from build123d import *

# Parameters (mm, degrees)
F0_W      = 31.75
F0_H      = 25.4
F0_R      = 3.175
F1_DEPTH  = 3.81
F2_W      = 31.75
F2_H      = 3.81
F3_DEPTH  = 25.4
F4_W      = 2.54
F4_H      = 25.4
F5_DEPTH  = 10.16
F4_W_2    = 8.89
F4_H_2    = 8.89
F6_DEPTH  = 25.4
F8_W      = 3.175
F8_H      = 25.4
F9_DEPTH  = 6.35
F7_W      = 3.18363
F7_H      = 25.4
F10_DEPTH = 6.35


with BuildPart() as f1:
    # F0 (on Top) → F1 (new body)
    with BuildSketch(Plane.XY):
        with Locations((-11.662145, 29.340504)):
            Rectangle(F0_W, F0_H)
        with Locations((-11.662145, 31.880504)):
            Circle(F0_R, mode=Mode.SUBTRACT)
    extrude(amount=F1_DEPTH)

    # F2 (on face) → F3 (join)
    with BuildSketch(Plane.XY.offset(3.81)):
        with Locations((-11.662145, 18.545504)):
            Rectangle(F2_W, F2_H)
    extrude(amount=F3_DEPTH)

    # F4 (on face) → F5 (join)
    with BuildSketch(Plane(origin=(0, 20.450504, 0), x_dir=(-1, 0, 0), z_dir=(0, 1, 0))):
        with Locations((-2.942855, 16.51)):
            Rectangle(F4_W, F4_H)
        with Locations((26.267145, 16.51)):
            Rectangle(F4_W, F4_H)
    extrude(amount=F5_DEPTH)

    # F4 (on face) → F6 (cut)
    with BuildSketch(Plane(origin=(0, 20.450504, 0), x_dir=(-1, 0, 0), z_dir=(0, 1, 0))):
        with Locations((11.662145, 18.415)):
            Rectangle(F4_W_2, F4_H_2)
    extrude(amount=-F6_DEPTH, mode=Mode.SUBTRACT)

    # F8 (on face) → F9 (join)
    with BuildSketch(Plane(origin=(1.672855, 0, 0), x_dir=(0, -1, 0), z_dir=(-1, 0, 0))):
        with Locations((-29.023004, 16.51)):
            Rectangle(F8_W, F8_H)
    extrude(amount=F9_DEPTH)

    # F7 (on face) → F10 (join)
    with BuildSketch(Plane.YZ.offset(-24.997145)):
        with Locations((29.018689, 16.51)):
            Rectangle(F7_W, F7_H)
    extrude(amount=F10_DEPTH)


solid = f1.part
Here's how the part is built. I have some questions about the finished solid (model axes, mm). A direction names the side the tool comes from. Round coordinates to 2 decimals unless told otherwise and drop trailing zeros. Loops run counter-clockwise (first coordinate to the right, second up) from the corner with the lowest first, then second, coordinate; pieces in that order, holes last.
1. If we section it at A-A on z = 17.5: Write out the boundary of the cut face in (x, y).
Answer list:
outline: (-27.54, 16.64) - (-16.11, 16.64) - (-16.11, 20.45) - (-25, 20.45) - (-25, 27.43) - (-18.65, 27.43) - (-18.65, 30.61) - (-27.54, 30.61) - close; (-7.22, 16.64) - (4.21, 16.64) - (4.21, 30.61) - (-4.68, 30.61) - (-4.68, 27.44) - (1.67, 27.44) - (1.67, 20.45) - (-7.22, 20.45) - close
2. Which directions (+Z, -Z, +X, -X, +Y, -Y) give clear straight access to the entire face, cutting with the end or side of a thin tool? Please do faces 1 (the face through (-1, 27.436, 16)), 2 (the face through (-23, 30.611, 16)), 3 (the face through (-12, 19, 22.86)), 4 (the face through (-4.677, 29, 17)).
Answer list:
face 1: +Z
face 2: +Z, +X, -X, +Y
face 3: +Y, -Y
face 4: +Z, +Y
3. If I drill on line 1 along X through (y, z) = (25.75, 9); line 2 along Y through (x, z) = (-0.5, 5); line 3 along Z through (x, y) = (-17, 24), over which ranges is the centre line in solid material (lowest first)?
Answer list:
line 1: x = -27.54 to -25, 1.67 to 4.21
line 2: y = 16.64 to 20.45, 27.44 to 30.61
line 3: z = 0 to 3.81
4. If we section it at C-C on x = -24.5: Write out the boundary of the cut face in (y, z), plus the area to 3 significant figures.
Answer list:
outline: (16.64, 0) - (42.04, 0) - (42.04, 3.81) - (30.61, 3.81) - (30.61, 29.21) - (27.43, 29.21) - (27.43, 3.81) - (20.45, 3.81) - (20.45, 29.21) - (16.64, 29.21) - close
area: 274 mm2
5. We'd pull the mould along X, two halves only. Please class faces 5 (the face through (4.213, 24, 14)), 6 (the face through (-12.075, 35.028, 1.878)), 7 (the face through (-27.537, 24, 14)), 8 (the face through (-12, 16.641, 11)): +X half, -X half, draft (parallel to the pull), parting line (faces both ways), or undercut.
Answer list:
face 5: +X half
face 6: undercut
face 7: -X half
face 8: draft
6. If we section it at B-B on y = 25.5: Write out the boundary of the cut face in (x, z).
Answer list:
outline: (-27.54, 0) - (4.21, 0) - (4.21, 29.21) - (1.67, 29.21) - (1.67, 3.81) - (-25, 3.81) - (-25, 29.21) - (-27.54, 29.21) - close
7. If we section it at D-D on z = 12.5: Write out the boundary of the cut face in (x, y).
Answer list:
outline: (-27.54, 16.64) - (4.21, 16.64) - (4.21, 30.61) - (-4.68, 30.61) - (-4.68, 27.44) - (1.67, 27.44) - (1.67, 20.45) - (-25, 20.45) - (-25, 27.43) - (-18.65, 27.43) - (-18.65, 30.61) - (-27.54, 30.61) - close
8. For P1, Ø2, axis at x = -9, y = 29.5, coming from the -Z side; P2, Ø3, axis at x = -22, z = 13, coming from the +Y side; P3, Ø1.5, axis at x = -3.5, y = 36.5, coming from the +Z side, each with a flat end and sliding along its axis, tell me the tip position at first contact or that it passes through.
Answer list:
P1: stops at z = 0
P2: stops at y = 30.61
P3: stops at z = 3.81
